Answer from the drawing. Dimensions are ordinates in mm from the lowest x, y and z of the part. A direction names the side the tool comes from. Coordinates: 2 decimals unless noted, no trailing zeros. Order: outer loops, then holes, each group sorted by start corner. A loop starts at its lowest first (then second) coordinate and runs counter-clockwise, first axis right, second up. Notation, with made-up numbers: (55, -21.75) - (81, -21.75) arc R23 ccw to (81, 0.25) - close; hole circle Ø11 at (22.5, 10). An arc over 180 degrees is marked (long way). Use a Markdown table: item, result. Add a question column.
Item 1: The part is cut by section C-C, the plane x = 20.75. Give the vertices of the cut face in (y, z), then the cut area to 3 significant figures.
Item 2: The part is cut by section B-B, the plane z = 12.5. Give the vertices of the cut face in (x, y).
Item 3: Flat-ended cylindrical pins translate along their axes: P1, Ø4, axis at x = 12.5, z = 3.75, coming from the +Y side; P2, Ø3, axis at x = 9, y = 7, coming from the +Z side; P3, Ø1.5, axis at x = 5, y = 12, coming from the +Z side; P4, Ø6, axis at x = 15.5, y = 13, coming from the -Z side. Find the tip coordinate at first contact, or state that the pin passes through.
Item 4: The part is cut by section A-A, the plane x = 12.5. Give the vertices of the cut face in (y, z), then the cut area to 3 significant figures.
Item 5: The part is cut by section D-D, the plane y = 2.25. Give the vertices of the cut face in (x, z).
Item 6: The mould has two halves that part along Y. Classify the marked faces 3, 4, 5 and 6: released by +Y, released by -Y, zero draft, split by the parting line, or undercut.
Item 7: For the marked faces 1 and 2, determine the directions among +Z, -Z, +X, -X, +Y, -Y from which every point of the face is accessible in a straight line to the end or side of a thin tool.
Item 8: Find the intervals of material crossed by line 1 along X through (y, z) = (3.75, 10.25); line 2 along Y through (x, z) = (18, 1.75); line 3 along X through (y, z) = (1.75, 21.25), in increasing order.
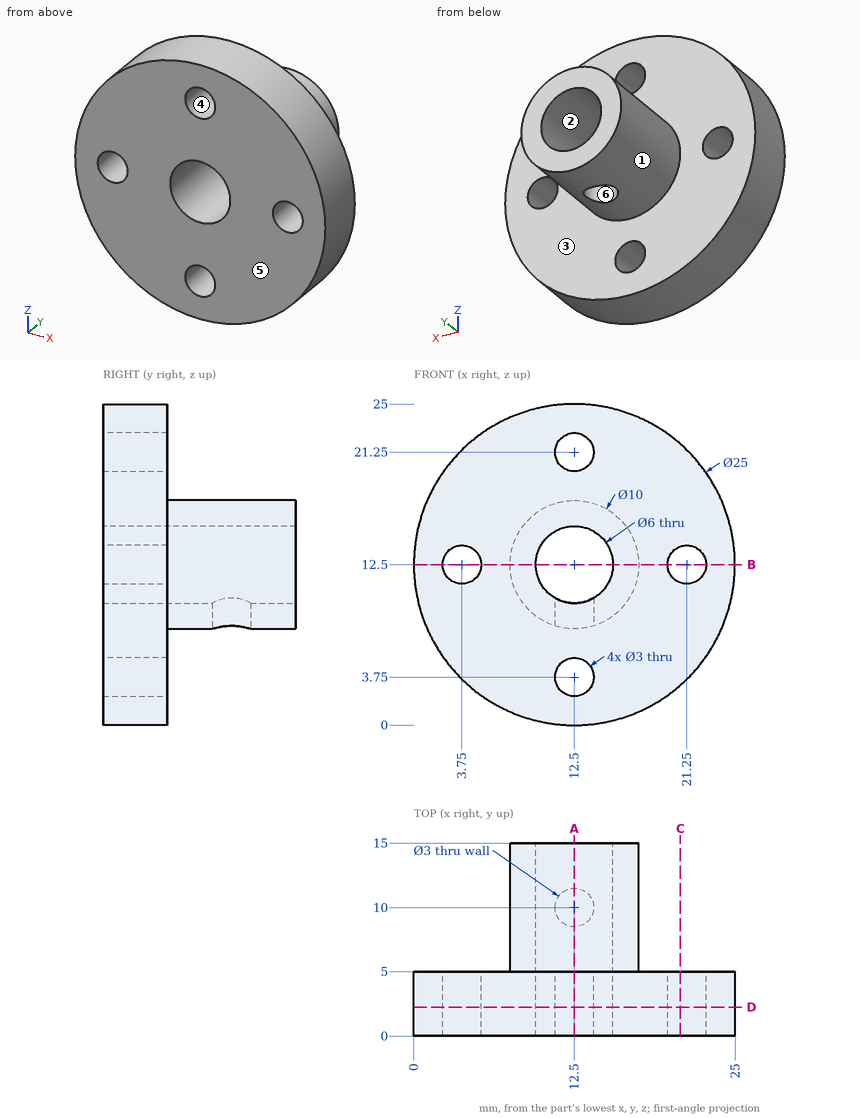
Solution:
| question | item | result |
|---|---|---|
| 1 | outline | (0, 3.11) - (5, 3.11) - (5, 11.09) - (0, 11.09) - close; (0, 13.91) - (5, 13.91) - (5, 21.89) - (0, 21.89) - close |
| 1 | area | 79.8 mm2 |
| 2 | outline | (0, 0) - (2.25, 0) - (2.25, 5) - (0, 5) - close; (5.25, 0) - (9.5, 0) - (9.5, 15) - (7.5, 15) - (7.5, 5) - (5.25, 5) - close; (15.5, 0) - (19.75, 0) - (19.75, 5) - (17.5, 5) - (17.5, 15) - (15.5, 15) - close; (22.75, 0) - (25, 0) - (25, 5) - (22.75, 5) - close |
| 3 | P1 | stops at y = 5 |
| 3 | P2 | stops at z = 17.08 |
| 3 | P3 | passes through |
| 3 | P4 | stops at z = 7.5 |
| 4 | outline | (0, 0) - (5, 0) - (5, 2.25) - (0, 2.25) - close; (0, 5.25) - (5, 5.25) - (5, 7.5) - (8.5, 7.5) - (8.5, 9.5) - (0, 9.5) - close; (0, 15.5) - (15, 15.5) - (15, 17.5) - (5, 17.5) - (5, 19.75) - (0, 19.75) - close; (0, 22.75) - (5, 22.75) - (5, 25) - (0, 25) - close; (11.5, 7.5) - (15, 7.5) - (15, 9.5) - (11.5, 9.5) - close |
| 4 | area | 99.0 mm2 |
| 5 | outline | circle Ø25 at (12.5, 12.5); hole circle Ø3 at (3.75, 12.5); hole circle Ø6 at (12.5, 12.5); hole circle Ø3 at (12.5, 3.75); hole circle Ø3 at (12.5, 21.25); hole circle Ø3 at (21.25, 12.5) |
| 6 | face 3 | released by +Y |
| 6 | face 4 | zero draft |
| 6 | face 5 | released by -Y |
| 6 | face 6 | undercut |
| 7 | face 1 | +Y |
| 7 | face 2 | +Y, -Y |
| 8 | line 1 | x = 0.2 to 10.52, 14.48 to 24.8 |
| 8 | line 2 | y = 0 to 5 |
| 8 | line 3 | x = 3.57 to 11, 14 to 21.43 |
